For this review, take the finished solid that the model builds, in its own axes (mm). A direction names the side the tool comes from. Coordinates: 2 decimals unless noted, no trailing zeros. Write each loop counter-clockwise with the first axis right and the second up, starting at its lowest first coordinate (ties: lowest second). Pieces come first, ordered by that corner, then holes. Notation, with made-up numbers: M -5,11.25 L 37,11.25 A12 cw 37,18.25 Z; hole C 53.5,88 d6. An arc over 180 degrees is marked long. One line per question, with ' | ' between items.
from build123d import *

# Parameters (mm, degrees)
BOSS_EXTRUDE1_DEPTH  = 50.8
SKETCH3_R            = 2.8575
CUT_EXTRUDE1_DEPTH   = 29.575
BOSS_EXTRUDE2_DEPTH  = 3.175
BOSS_EXTRUDE4_DEPTH  = 50.8
CUT_EXTRUDE2_REACH   = 108.711
BOSS_EXTRUDE5_DEPTH  = 8.255
BOSS_EXTRUDE6_REACH  = 116.966
CUT_EXTRUDE3_DEPTH   = 8.255
BOSS_EXTRUDE10_DEPTH = 3.175
BOSS_EXTRUDE11_DEPTH = 8.255
CUT_EXTRUDE4_START   = -11.43
CUT_EXTRUDE4_DEPTH   = 8.255
BOSS_EXTRUDE12_DEPTH = 4.445
CUT_EXTRUDE5_DEPTH   = 4.445
BOSS_EXTRUDE13_START = -50.8
BOSS_EXTRUDE13_DEPTH = 4.445
CUT_EXTRUDE6_START   = -50.8
CUT_EXTRUDE6_DEPTH   = 4.445
SKETCH18_R           = 5.08
CUT_EXTRUDE7_DEPTH   = 55.801163899


with BuildPart() as part:
    # Sketch2 → Boss-Extrude1 (new body)
    with BuildSketch(Plane(origin=(0, 0, 0), x_dir=(0, 0, -1), z_dir=(1, 0, 0))):
        Polygon((0, 0), (31.75, 0), (31.75, -28.575), (28.575, -28.575), (28.575, -3.175), (3.175, -3.175), (3.175, -28.575), (0, -28.575), align=None)
    extrude(amount=BOSS_EXTRUDE1_DEPTH)

    # Sketch3 → Cut-Extrude1 (cut, through all)
    with BuildSketch(Plane(origin=(0, 0, 0), x_dir=(1, 0, 0), z_dir=(0, 1, 0))):
        with Locations((12.7, 15.875)):
            Circle(SKETCH3_R)
        with Locations((38.1, 15.875)):
            Circle(SKETCH3_R)
    extrude(amount=-CUT_EXTRUDE1_DEPTH, mode=Mode.SUBTRACT)

    # Sketch4 → Boss-Extrude2 (add)
    with BuildSketch(Plane(origin=(0, 0, 0), x_dir=(1, 0, 0), z_dir=(0, 1, 0))):
        Polygon((0, 31.75), (76.2, 75.744090512), (101.6, 31.75), (50.8, 2.420606325), (50.8, 31.75), align=None)
    extrude(amount=-BOSS_EXTRUDE2_DEPTH)

    # Sketch6 → Boss-Extrude4 (add)
    with BuildSketch(Plane(origin=(-13.748153285, 0, -23.8125), x_dir=(-0.866025404, 0, 0.5), z_dir=(-0.5, 0, -0.866025404))):
        Polygon((-103.863181024, -3.175), (-128.994432583, 32.716146821), (-126.393624843, 34.537252006), (-102.210380639, 0), (-103.863181024, 0), align=None)
    extrude(amount=-BOSS_EXTRUDE4_DEPTH)

    # Sketch7 → Cut-Extrude2 (cut, up to next)
    with BuildSketch(Plane(origin=(61.648020601, -49.844275413, -35.592501289), x_dir=(-0.318495595, 0.25751325, -0.91227599), z_dir=(0.70940648, -0.573576436, -0.409576022)), mode=Mode.PRIVATE) as cut_extrude2_sk1:
        Polygon((20.449889648, 80.334208308), (35.520058582, 75.3436539), (33.124592466, 68.109972811), (18.054423532, 73.100527219), align=None)
    cut_extrude2_tool1 = extrude(cut_extrude2_sk1.sketch, amount=-CUT_EXTRUDE2_REACH, mode=Mode.PRIVATE) & part.part
    add(cut_extrude2_tool1.solids().sort_by_distance((99.782151, 14.770573, -60.029858))[0], mode=Mode.SUBTRACT)
    # Sketch7 → Cut-Extrude2 (cut, up to next)
    with BuildSketch(Plane(origin=(61.648020601, -49.844275413, -35.592501289), x_dir=(-0.318495595, 0.25751325, -0.91227599), z_dir=(0.70940648, -0.573576436, -0.409576022)), mode=Mode.PRIVATE) as cut_extrude2_sk2:
        Polygon((7.213752471, 71.673620272), (40.970930883, 60.494778398), (39.373953472, 55.672324339), (5.61677506, 66.851166213), align=None)
    cut_extrude2_tool2 = extrude(cut_extrude2_sk2.sketch, amount=-CUT_EXTRUDE2_REACH, mode=Mode.PRIVATE) & part.part
    add(cut_extrude2_tool2.solids().sort_by_distance((94.262219, 5.667746, -56.842924))[0], mode=Mode.SUBTRACT)

    # Sketch8 → Boss-Extrude5 (add)
    with BuildSketch(Plane(origin=(61.648020601, -49.844275413, -35.592501289), x_dir=(-0.318495595, 0.25751325, -0.91227599), z_dir=(0.70940648, -0.573576436, -0.409576022))):
        Polygon((-4.21199432, 61.410144483), (44.012546269, 45.440370378), (57.786476434, 87.034036636), (9.561935845, 103.003810741), align=None)
        Polygon((11.577858751, 98.991666073), (-0.199849652, 63.426067388), (41.996623363, 49.452515046), (53.774331766, 85.018113731), align=None, mode=Mode.SUBTRACT)
    extrude(amount=BOSS_EXTRUDE5_DEPTH)

    # Boss-Extrude6: up to this face of the body (flat: up to its plane)
    boss_extrude6_end = Plane(part.part.faces().sort_by_distance((50.815624122, -3.175, -33.129894289))[0])
    # Sketch9 → Boss-Extrude6 (add, up to the picked face)
    with BuildSketch(Plane(origin=(67.504171093, -54.579148895, -38.973551352), x_dir=(-0.318495595, 0.25751325, -0.91227599), z_dir=(0.70940648, -0.573576436, -0.409576022)), mode=Mode.PRIVATE) as boss_extrude6_sk1:
        Polygon((0.007652981, 60.012789249), (39.792898967, 46.837725612), (38.994410262, 44.426498583), (-0.790835724, 57.601562219), align=None)
    boss_extrude6_tool1 = split(extrude(boss_extrude6_sk1.sketch, amount=-BOSS_EXTRUDE6_REACH, mode=Mode.PRIVATE), bisect_by=boss_extrude6_end, keep=Keep.BOTH, mode=Mode.PRIVATE)
    add(boss_extrude6_tool1.solids().sort_by_distance((94.125301, -8.950197, -56.763874))[0])

    # Sketch10 → Cut-Extrude3 (cut)
    with BuildSketch(Plane(origin=(67.504171093, -54.579148895, -38.973551352), x_dir=(-0.318495595, 0.25751325, -0.91227599), z_dir=(0.70940648, -0.573576436, -0.409576022))):
        Polygon((4.019797649, 62.028712154), (37.776976062, 50.84987028), (36.978487357, 48.438643251), (3.221308944, 59.617485125), align=None)
    extrude(amount=-CUT_EXTRUDE3_DEPTH, mode=Mode.SUBTRACT)

    # Sketch14 → Boss-Extrude10 (add)
    with BuildSketch(Plane(origin=(67.504171093, -54.579148895, -38.973551352), x_dir=(-0.318495595, 0.25751325, -0.91227599), z_dir=(0.70940648, -0.573576436, -0.409576022))):
        Polygon((-2.515205822, 66.534001921), (-7.337659881, 68.130979331), (-3.744460707, 78.981500964), (1.077993352, 77.384523553), (0.07988247, 74.370489766), (-1.728537802, 74.969356295), (-3.325515212, 70.146902236), (-1.51709494, 69.548035707), align=None)
        Polygon((5.058616193, 95.464786046), (6.867036465, 94.865919517), (7.865147347, 97.879953304), (3.042693288, 99.476930714), (-0.550505886, 88.626409082), (4.271948173, 87.029431671), (5.270059055, 90.043465458), (3.461638782, 90.642331987), align=None)
        Polygon((55.303019916, 73.474824824), (56.899997326, 78.297278883), (55.091577054, 78.896145411), (56.089687936, 81.910179198), (60.912141995, 80.313201788), (57.318942821, 69.462680155), (52.496488762, 71.059657566), (53.494599644, 74.073691353), align=None)
        Polygon((48.515865921, 52.979395073), (46.707445649, 53.578261602), (45.709334767, 50.564227815), (50.531788826, 48.967250405), (54.124988, 59.817772037), (49.302533941, 61.414749448), (48.304423059, 58.400715661), (50.112843331, 57.801849132), align=None)
    extrude(amount=-BOSS_EXTRUDE10_DEPTH)

    # Sketch15 → Boss-Extrude11 (add)
    with BuildSketch(Plane(origin=(61.648020601, -49.844275413, -35.592501289), x_dir=(-0.318495595, 0.25751325, -0.91227599), z_dir=(0.70940648, -0.573576436, -0.409576022))):
        Polygon((4.019797649, 62.028712154), (7.213752471, 71.673620272), (40.970930883, 60.494778398), (37.776976062, 50.84987028), (41.996623363, 49.452515046), (53.774331766, 85.018113731), (11.577858751, 98.991666073), (-0.199849652, 63.426067388), align=None)
        Polygon((20.449889648, 80.334208308), (35.520058582, 75.3436539), (33.124592466, 68.109972811), (18.054423532, 73.100527219), align=None, mode=Mode.SUBTRACT)
    extrude(amount=BOSS_EXTRUDE11_DEPTH)

    # Sketch16 → Cut-Extrude4 (cut)
    with BuildSketch(Plane(origin=(67.504171093, -54.579148895, -38.973551352), x_dir=(-0.318495595, 0.25751325, -0.91227599), z_dir=(0.70940648, -0.573576436, -0.409576022)).offset(CUT_EXTRUDE4_START)):
        Polygon((9.561935845, 103.003810741), (-3.213883439, 64.42417827), (1.005763863, 63.026823036), (5.197829565, 75.68576494), (44.983075551, 62.510701303), (40.791009849, 49.851759399), (45.01065715, 48.454404165), (57.786476434, 87.034036636), align=None)
    extrude(amount=CUT_EXTRUDE4_DEPTH, mode=Mode.SUBTRACT)

    # Sketch17 → Boss-Extrude12 (add)
    with BuildSketch(Plane(origin=(11.651846715, 0, 20.181590512), x_dir=(0.866025404, 0, -0.5), z_dir=(0.5, 0, 0.866025404))):
        Polygon((111.120352225, -1.667395138), (112.287874869, 0), (104.864254679, 0), (109.845578595, -3.487960556), align=None)
    extrude(amount=-BOSS_EXTRUDE12_DEPTH)

    # Sketch17<3> → Cut-Extrude5 (cut)
    with BuildSketch(Plane(origin=(11.651846715, 0, 20.181590512), x_dir=(0.866025404, 0, -0.5), z_dir=(0.5, 0, 0.866025404))):
        Polygon((102.210380639, 0), (104.864254679, 0), (103.083478469, 1.246912926), align=None)
    extrude(amount=-CUT_EXTRUDE5_DEPTH, mode=Mode.SUBTRACT)

    # Sketch17<4> → Boss-Extrude13 (add)
    with BuildSketch(Plane(origin=(11.651846715, 0, 20.181590512), x_dir=(0.866025404, 0, -0.5), z_dir=(0.5, 0, 0.866025404)).offset(BOSS_EXTRUDE13_START)):
        Polygon((111.120352225, -1.667395138), (112.287874869, 0), (104.864254679, 0), (109.845578595, -3.487960556), align=None)
    extrude(amount=BOSS_EXTRUDE13_DEPTH)

    # Sketch17<5> → Cut-Extrude6 (cut)
    with BuildSketch(Plane(origin=(11.651846715, 0, 20.181590512), x_dir=(0.866025404, 0, -0.5), z_dir=(0.5, 0, 0.866025404)).offset(CUT_EXTRUDE6_START)):
        Polygon((102.210380639, 0), (104.864254679, 0), (103.083478469, 1.246912926), align=None)
    extrude(amount=CUT_EXTRUDE6_DEPTH, mode=Mode.SUBTRACT)

    # Sketch18 → Cut-Extrude7 (cut, through all)
    with BuildSketch(Plane(origin=(65.251805519, -52.758043709, -37.673147481), x_dir=(0.318495595, -0.25751325, 0.91227599), z_dir=(-0.70940648, 0.573576436, 0.409576022))):
        with Locations((-26.787241057, 74.222090559)):
            Circle(SKETCH18_R)
    extrude(amount=-CUT_EXTRUDE7_DEPTH, mode=Mode.SUBTRACT)


solid = part.part
1) The part is to be moulded in two halves that separate along X. For faces 4 (the flat face through (100.55, 11, -69.64)), 5 (the flat face through (25, -28.575, -2)), 6 (the cylindrical face through (101.947, 6.798, -61.339)), 7 (the flat face through (87.26, 4.17, -83.21)), say which applies: +X half, -X half, draft (parallel to the pull), parting line (faces both ways), or undercut.
Responses:
face 4: undercut | face 5: draft | face 6: +X half | face 7: undercut
2) We need section D-D on x = 70.5. State the section outline as (y, z) points (3 decimals).
Responses:
outline: M -3.175,-72.453 L 0,-72.453 L 0,-13.794 L -3.175,-13.794 Z
3) Machinability: for faces 1 (the flat face through (110.28, -2.59, -33.87)), 2 (the flat face through (105.41, 7.84, -56.79)), 3 (the flat face through (126.8, 26.7, -46.3)), which of the approach directions +Z, -Z, +X, -X, +Y, -Y give a long, thin tool a straight path to every point of the face, cutting with its end or side? Answer none if there is none.
Responses:
face 1: +Z, -Y | face 2: -Z, +Y | face 3: +X, +Y
4) To check wall thickness, follow line 1 along Y through (x, z) = (70, -66) (3 decimals); line 2 along Z through (x, y) = (38.1, -1); line 3 along Z through (x, y) = (12.7, -2.4). State the ranges of each line that lie inside material, in increasing order. Write a range as [from, to].
Responses:
line 1: [-3.175, 0] | line 2: [-53.75, -18.73], [-13.02, 0] | line 3: [-39.08, -18.73], [-13.02, 0]
5) Insertion check: pin 1 Ø6 at (y, z) = (14.5, -68.5) entering from -X; pin 2 Ø4.5 at (x, z) = (12.7, -15.875) entering from +Y; pin 3 Ø8 at (y, z) = (1, -38) entering from +X; pin 4 Ø6.5 at (x, z) = (38.1, -15.875) entering from +Y. Each pin has a flat end and moves straight along its axis. Give the tip position at first contact, or say it passes through.
Responses:
pin 1: x = 87.22 | pin 2: through | pin 3: x = 116.98 | pin 4: y = 0
6) We need section C-C on z = -21. State the section outline as (x, y) points (3 decimals).
Responses:
outline: M 0,-3.175 L 82.98,-3.175 L 82.98,0 L 0,0 Z
